Autodesk Fusion 360 part; units mm, degrees
sketch "Sketch1" plane through (0, 0, 0) normal (0, 1, 0) x (1, 0, 0)
  line L0 (12, 3.2) -> (12, 0)
  line L1 (12, 0) -> (0, 0)
  line L2 (-18, -3.2) -> (-18, 0)
  circle A0 centre (-15.5, -3.2) radius 1.05
  line L3 (-7.0785, 3.2) -> (-8, 0)
  line L4 (-8, 0) -> (-18, 0)
  line L5 (-7.0785, 3.2) -> (12, 3.2)
  line L6 (-3.8, 2.1) -> (-3.8, -2.1)
  line L7 (-3.8, -2.1) -> (-2, -2.1)
  line L8 (-2, -2.1) -> (-2, 2.1)
  line L9 (-2, 2.1) -> (-3.8, 2.1)
  line L10 (0, -3.2) -> (-13, -3.2)
  line L11 (0, -3.2) -> (0, 0)
  arc A1 (-18, -3.2) -> (-13, -3.2) centre (-15.5, -3.2) ccw
  dimension "d9" = 2.1
  dimension "d15" = 3.2
  dimension "d22" = 10
  dimension "d23" = 4.2
  dimension "d24" = 1.8
  dimension "d35" = 12
  dimension "d37" = 2.5
  dimension "d39" = 3.2
  dimension "d40" = 18
  dimension "d42" = 5
  dimension "d43" = 3.2
  dimension "d50" = 2
extrude "Extrude2" add sketch "Sketch1" along normal blind 3.2
sketch "Sketch3" plane through (-18, 0, 0) normal (-1, 0, 0) x (0, 0, 1)
  line L0 (0, 0) -> (3.2, 0)
  line L1 (3.2, 0) -> (3.2, 3.2)
  line L2 (3.2, 3.2) -> (0, 3.2)
  line L3 (0, 3.2) -> (0, 0)
  circle A0 centre (0, 1.6) radius 1
  circle A1 centre (0, 1.6) radius 2
  dimension "d44" = 2
  dimension "d45" = 4
extrude "Extrude7" cut sketch "Sketch3" against normal blind 30 contours L3 A0 | L3 A0
extrude "Extrude8" cut sketch "Sketch3" against normal blind 12 contours L0 L2 L3 A0 A1 | L0 L2 L3 A0 A1
fillet "Fillet4" radius 1 1 edges at (-13, 1.6, 3.2)
Here's how the part is built. I have some questions about the finished solid (model axes, mm). A direction names the side the tool comes from. Coordinates: 2 decimals unless noted, no trailing zeros. Order: outer loops, then holes, each group sorted by start corner. A loop starts at its lowest first (then second) coordinate and runs counter-clockwise, first axis right, second up. Notation, with made-up numbers: M 7,-3.75 L 44,-3.75 A22 ccw 44,31.25 Z; hole C -3.75,83 d3. An arc over 180 degrees is marked long. Answer as CSV lines item,"result".
Item 1: We'd pull the mould along Y, two halves only. Please class faces 4 (the face through (-12.1, 1.6, 2)), 5 (the face through (-4, 0, 0)), 6 (the face through (-4, 3.2, 0)): +Y half, -Y half, draft (parallel to the pull), parting line (faces both ways), or undercut.
Results found:
face 4,"undercut"
face 5,"-Y half"
face 6,"+Y half"
Item 2: Imagine slicing it at C-C on x = -4.75. Write out the boundary of the cut face in (y, z).
Results found:
outline,"M 0,-3.2 L 3.2,-3.2 L 3.2,3.2 L 0,3.2 Z; hole C 1.6,0 d2"
Item 3: Imagine slicing it at B-B on y = 1.1. Write out the boundary of the cut face in (x, z).
Results found:
outline,"M -18,1.94 L -6,1.94 L -6,0.87 L -3.8,0.87 L -3.8,2.1 L -2,2.1 L -2,0.87 L 0,0.87 L 0,3.2 L -12.15,3.2 A1 cw -13.1,3.91 A2.5 ccw -18,3.2 Z; M -7.44,-1.94 L -7.08,-3.2 L 12,-3.2 L 12,-0.87 L -2,-0.87 L -2,-2.1 L -3.8,-2.1 L -3.8,-0.87 L -6,-0.87 L -6,-1.94 Z; hole C -15.5,3.2 d2.1"
Item 4: For pin 1 (1 mm diameter, centred on y = 1, z = 1, fed in from -X); pin 2 (1.6 mm diameter, centred on y = 2, z = 2, fed in from +X); pin 3 (0.5 mm diameter, centred on x = -3, y = 1.5, fed in from +Z), each with a flat end and sliding along its axis, tell me the tip position at first contact or that it passes through.
Results found:
pin 1,"x = -6"
pin 2,"x = 0"
pin 3,"z = 3.2"
Item 5: Imagine slicing it at D-D on z = 2.5. Write out the boundary of the cut face in (x, y).
Results found:
outline,"M -18,0 L -16.28,0 L -16.28,3.2 L -18,3.2 Z; M -14.72,0 L 0,0 L 0,3.2 L -14.72,3.2 Z"
Item 6: Imagine slicing it at A-A on x = -15.5. Write out the boundary of the cut face in (y, z).
Results found:
outline,"M 0,1.2 A2 cw 3.2,1.2 L 3.2,2.15 L 0,2.15 Z; M 0,4.25 L 3.2,4.25 L 3.2,5.7 L 0,5.7 Z"
Item 7: On a 3-axis mill with a long thin cutter (end or side, diameter ignored), from which of +Z, -Z, +X, -X, +Y, -Y can I reach the whole of each face in a straight line? I mean faces 1 (the face through (-3.8, 1, -1)), 2 (the face through (-6, 3, 0)), 3 (the face through (0, 2, 2)). Say none if no direction works.
Results found:
face 1,"+Y, -Y"
face 2,"-X"
face 3,"+Z, +X, +Y, -Y"
Item 8: If I drill on line 1 (X direction, y = 0.85, z = 0.75); line 2 (Z direction, x = -5.4, y = 1.6); line 3 (X direction, y = 0.45, z = -0.75), over which ranges is the centre line in solid material (lowest first)?
Results found:
line 1,"-6 to -3.8, -2 to 0"
line 2,"-3.2 to -1, 1 to 3.2"
line 3,"-6 to -3.8, -2 to 12"
